Read the model definition and answer for the solid it produces. Units are mm, in the model's axes. Face numbers are marked on the shaded views. A direction names the side the tool comes from. Give positions to 0.01 mm unless a question says otherwise; leave off trailing zeros. Order: outer loops, then holes, each group sorted by start corner. A loop starts at its lowest first (then second) coordinate and runs counter-clockwise, first axis right, second up. Notation, with made-up numbers: M 46.5,41 L 90.5,41 A9 cw 90.5,45 Z; hole C 62.5,65.5 d5. An arc over 180 degrees is marked long. One line per item, written item: value.
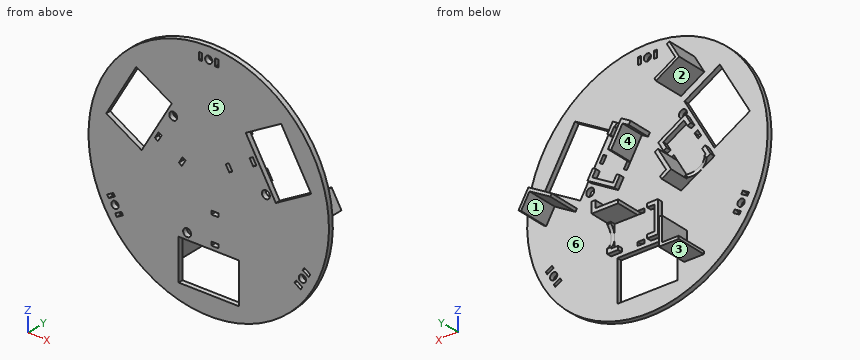
from build123d import *

# Parameters (mm, degrees)
SKETCH_1_R               = 50
SKETCH_1_W               = 25
SKETCH_1_H               = 17
EXTRUDE_1_DEPTH          = 2
EXTRUDE_2_DEPTH          = 2
SKETCH_3_R               = 6.1
CUT_EXTRUDE_1_DEPTH      = 3
SKETCH_4_W               = 3
SKETCH_4_H               = 1.5
CUT_EXTRUDE_2_DEPTH      = 3
PATTERN_CIRCULAR_2_COUNT = 3
SKETCH_5_R               = 1.5
SKETCH_5_W               = 1.3
SKETCH_5_H               = 3
CUT_EXTRUDE_3_DEPTH      = 3
PATTERN_CIRCULAR_3_COUNT = 3
EXTRUDE_3_DEPTH          = 10
PATTERN_CIRCULAR_6_COUNT = 3
EXTRUDE_4_DEPTH          = 13
PATTERN_CIRCULAR_7_COUNT = 3
SKETCH_10_R              = 1.65
CUT_EXTRUDE_4_DEPTH      = 8
PATTERN_CIRCULAR_8_COUNT = 3


with BuildPart() as part:
    # 草图1 → 凸台-拉伸1 (new body)
    with BuildSketch(Plane(origin=(0, 0, 0), x_dir=(1, 0, 0), z_dir=(0, 1, 0))):
        with Locations(Location((0, 0, 0), (0, 0, 270))):
            Circle(SKETCH_1_R)
        Polygon((42.623066959, -10.174682453), (27.900635095, -1.674682453), (15.400635095, -23.325317547), (30.123066959, -31.825317547), align=None, mode=Mode.SUBTRACT)
        with Locations((0, 33.5)):
            Rectangle(SKETCH_1_W, SKETCH_1_H, mode=Mode.SUBTRACT)
        Polygon((-30.123066959, -31.825317547), (-15.400635095, -23.325317547), (-27.900635095, -1.674682453), (-42.623066959, -10.174682453), align=None, mode=Mode.SUBTRACT)
    extrude(amount=-EXTRUDE_1_DEPTH)

    # 草图2 → 凸台-拉伸2 (add)
    with BuildSketch(Plane(origin=(0, 0, 0), x_dir=(1, 0, 0), z_dir=(0, 1, 0))):
        Polygon((10.6, 23.5), (10.6, 22), (13.6, 22), (13.6, 12), (10.6, 12), (10.6, 10.5), (15.1, 10.5), (15.1, 23.5), align=None)
        Polygon((-4.5, 12), (-4.5, 22), (-1.5, 22), (-1.5, 23.5), (-6, 23.5), (-6, 10.5), (-1.5, 10.5), (-1.5, 12), align=None)
    extrude_2 = extrude(amount=EXTRUDE_2_DEPTH)

    # 草图3 → 切除-拉伸1 (cut)
    with BuildSketch(Plane(origin=(15.1, 0, 0), x_dir=(0, 0, -1), z_dir=(1, 0, 0))):
        with Locations((17, 6.1)):
            Circle(SKETCH_3_R)
    cut_extrude_1 = extrude(amount=-CUT_EXTRUDE_1_DEPTH, mode=Mode.SUBTRACT)

    # 草图4 → 切除-拉伸2 (cut)
    with BuildSketch(Plane(origin=(0, 0, 0), x_dir=(1, 0, 0), z_dir=(0, 1, 0))):
        with Locations((2.6, 22.75)):
            Rectangle(SKETCH_4_W, SKETCH_4_H)
        with Locations((2.6, 11.25)):
            Rectangle(SKETCH_4_W, SKETCH_4_H)
    cut_extrude_2 = extrude(amount=-CUT_EXTRUDE_2_DEPTH, mode=Mode.SUBTRACT)

    # 阵列(圆周)2: 凸台-拉伸2, 切除-拉伸1, 切除-拉伸2 ×3 about axis
    pattern_circular_2_axis = Axis((0, 0, 0), (0, 1, 0))
    add([extrude_2.rotate(pattern_circular_2_axis, i * 360 / PATTERN_CIRCULAR_2_COUNT) for i in range(1, PATTERN_CIRCULAR_2_COUNT)])
    add([cut_extrude_1.rotate(pattern_circular_2_axis, i * 360 / PATTERN_CIRCULAR_2_COUNT) for i in range(1, PATTERN_CIRCULAR_2_COUNT)], mode=Mode.SUBTRACT)
    add([cut_extrude_2.rotate(pattern_circular_2_axis, i * 360 / PATTERN_CIRCULAR_2_COUNT) for i in range(1, PATTERN_CIRCULAR_2_COUNT)], mode=Mode.SUBTRACT)

    # 草图5 → 切除-拉伸3 (cut)
    with BuildSketch(Plane(origin=(0, 0, 0), x_dir=(1, 0, 0), z_dir=(0, 1, 0))):
        with Locations(Location((0, -45, 0), (0, 0, 270))):
            Circle(SKETCH_5_R)
        with Locations((-3.35, -45)):
            Rectangle(SKETCH_5_W, SKETCH_5_H)
        with Locations((3.35, -45)):
            Rectangle(SKETCH_5_W, SKETCH_5_H)
    cut_extrude_3 = extrude(amount=-CUT_EXTRUDE_3_DEPTH, mode=Mode.SUBTRACT)

    # 阵列(圆周)3: 切除-拉伸3 ×3 about axis
    pattern_circular_3_axis = Axis((0, 0, 0), (0, 1, 0))
    for i in range(1, PATTERN_CIRCULAR_3_COUNT):
        add(cut_extrude_3.rotate(pattern_circular_3_axis, i * 360 / PATTERN_CIRCULAR_3_COUNT), mode=Mode.SUBTRACT)

    # 草图8 → 凸台-拉伸3 (add)
    with BuildSketch(Plane(origin=(0, 0, 0), x_dir=(1, 0, 0), z_dir=(0, 1, 0))):
        Polygon((4.1, 12), (15.1, 12), (15.1, 10.5), (15.1, 7.5), (13.6, 7.5), (13.6, 10.5), (4.1, 10.5), align=None)
    extrude_3 = extrude(amount=EXTRUDE_3_DEPTH)

    # 阵列(圆周)6: 凸台-拉伸3 ×3 about axis
    pattern_circular_6_axis = Axis((0, 0, 0), (0, 1, 0))
    for i in range(1, PATTERN_CIRCULAR_6_COUNT):
        add(extrude_3.rotate(pattern_circular_6_axis, i * 360 / PATTERN_CIRCULAR_6_COUNT))

    # 草图9 → 凸台-拉伸4 (add)
    with BuildSketch(Plane(origin=(0, 0, 0), x_dir=(1, 0, 0), z_dir=(0, 1, 0))):
        Polygon((-16.5, 35), (-16.5, 25), (-15.3, 25), (-15.3, 36.2), (-23.5, 36.2), (-23.5, 35), align=None)
    extrude_4 = extrude(amount=EXTRUDE_4_DEPTH)

    # 阵列(圆周)7: 凸台-拉伸4 ×3 about axis
    pattern_circular_7_axis = Axis((0, 0, 0), (0, 1, 0))
    for i in range(1, PATTERN_CIRCULAR_7_COUNT):
        add(extrude_4.rotate(pattern_circular_7_axis, i * 360 / PATTERN_CIRCULAR_7_COUNT))

    # 草图10 → 切除-拉伸4 (cut)
    with BuildSketch(Plane(origin=(0, 0, 0), x_dir=(1, 0, 0), z_dir=(0, 1, 0))):
        with Locations(Location((23.767848868, -3.330069097, 0), (0, 0, 270))):
            Circle(SKETCH_10_R)
    cut_extrude_4 = extrude(amount=-CUT_EXTRUDE_4_DEPTH, mode=Mode.SUBTRACT)

    # 阵列(圆周)8: 切除-拉伸4 ×3 about axis
    pattern_circular_8_axis = Axis((0, 0, 0), (0, 1, 0))
    for i in range(1, PATTERN_CIRCULAR_8_COUNT):
        add(cut_extrude_4.rotate(pattern_circular_8_axis, i * 360 / PATTERN_CIRCULAR_8_COUNT), mode=Mode.SUBTRACT)


solid = part.part
1) Find section A-A, the plane z = -39. Write down the section's boundary in (x, y), plus the area to 3 significant figures.
Reported:
outline: M -31.29,-2 L -12.5,-2 L -12.5,0 L -31.29,0 Z; M 12.5,-2 L 31.29,-2 L 31.29,0 L 12.5,0 Z
area: 75.2 mm^2
2) Find section C-C, the plane z = 45. Write down the section's boundary in (x, y), plus the area to 3 significant figures.
Reported:
outline: M -21.79,-2 L -4,-2 L -4,0 L -21.79,0 Z; M -2.7,-2 L -1.5,-2 L -1.5,0 L -2.7,0 Z; M 1.5,-2 L 2.7,-2 L 2.7,0 L 1.5,0 Z; M 4,-2 L 21.79,-2 L 21.79,0 L 4,0 Z
area: 76.0 mm^2
3) Find section B-B, the plane y = 5. Count the separate pieces of the cut face and the enclosed holes in it, plus the area to 3 significant figures.
Reported:
separate pieces: 6
enclosed holes: 0
area: 129 mm^2
4) Which of the six approach directions +Z, -Z, +X, -X, +Y, -Y give full straight-line access (tool end or side, diameter ignored) to the marked faces 1 and 2?
Reported:
face 1: -Z, +Y
face 2: -X, +Y
5) Determine the mould class of the marked faces 3, 4, 5 and 6 for opening direction Z: +Z half, -Z half, draft (parallel to the pull), parting line (faces both ways), or undercut.
Reported:
face 3: -Z half
face 4: undercut
face 5: draft
face 6: undercut
6) Consider probe 1 along Z at (x, y) = (6, 3); probe 2 along X at (y, z) = (-1.35, 45); probe 3 along Z at (x, y) = (-15, 0.5). Determine where each line is inside the solid, lowest interval first.
Reported:
probe 1: z = -12 to -10.5, 10.61 to 13.61
probe 2: x = -21.79 to -4, -2.7 to -1.5, 1.5 to 2.7, 4 to 21.79
probe 3: z = -8.78 to -7.04, -4.98 to -1.98, 13.86 to 15.59, 26.33 to 27.71
7) Each of these flat-tipped pins is pushed along its axis until it touches: pin 1 Ø4 at (y, z) = (8, -9) entering from -X; pin 2 Ø2 at (y, z) = (-1.5, 45) entering from +X; pin 3 Ø1 at (x, y) = (-4.5, 1.5) entering from +Z. Where does it stop, or does it pass through?
Reported:
pin 1: stops at x = -17.94
pin 2: stops at x = 23.75
pin 3: stops at z = -10.5
